```python
from build123d import *

# Parameters (mm, degrees)
SKETCH1_R                      = 6.35
SKETCH1_R_2                    = 5.08
BOSS_EXTRUDE1_DEPTH            = 15.494
BOSS_EXTRUDE2_DEPTH            = 13.462
SKETCH3_W                      = 1.016
SKETCH3_H                      = 0.508
BOSS_EXTRUDE3_DEPTH            = 1.27
SKETCH7_R                      = 1.397
CUT_EXTRUDE1_DEPTH             = 20.32
CUT_EXTRUDE4_REACH             = 23.971
CUT_EXTRUDE4_END_RADIUS        = 5.08
CUT_EXTRUDE4_DIRECTION_2_DEPTH = 0.635


with BuildPart() as part:
    # Sketch1 → Boss-Extrude1 (new body)
    with BuildSketch(Plane(origin=(0, 0, 0), x_dir=(0, 0, -1), z_dir=(1, 0, 0))):
        Circle(SKETCH1_R)
        Circle(SKETCH1_R_2, mode=Mode.SUBTRACT)
    extrude(amount=BOSS_EXTRUDE1_DEPTH)

    # Sketch2 → Boss-Extrude2 (add)
    with BuildSketch(Plane(origin=(1.016, 0, 0), x_dir=(0, 0, -1), z_dir=(1, 0, 0))):
        with BuildLine():
            Line((-2.0066, 6.024620854), (-2.0066, 14.224))
            Line((-2.0066, 14.224), (2.0066, 14.224))
            Line((2.0066, 14.224), (2.0066, 6.024620854))
            ThreePointArc((2.0066, 6.024620854), (0, 6.35), (-2.0066, 6.024620854))
        make_face()
    extrude(amount=BOSS_EXTRUDE2_DEPTH)

    # Sketch3 → Cut-Revolve1 (revolve, cut)
    with BuildSketch(Plane.XY, mode=Mode.PRIVATE) as cut_revolve1_sk:
        with Locations((14.986, 6.096)):
            Rectangle(SKETCH3_W, SKETCH3_H)
        with Locations((0.508, 6.096)):
            Rectangle(SKETCH3_W, SKETCH3_H)
    revolve(cut_revolve1_sk.sketch.rotate(Axis((15.494, 0, 0), (-1, 0, 0)), 90), axis=Axis((15.494, 0, 0), (-1, 0, 0)), mode=Mode.SUBTRACT)

    # Sketch5 → Boss-Extrude3 (add)
    with BuildSketch(Plane.ZY):
        with BuildLine():
            Line((4.709286039, 0.635), (4.709286039, -1.905))
            ThreePointArc((4.709286039, -1.905), (5.037440444, -0.656196444), (5.040156248, 0.635))
            Line((5.040156248, 0.635), (4.709286039, 0.635))
        make_face()
    extrude(amount=-BOSS_EXTRUDE3_DEPTH)

    # Sketch7 → Cut-Extrude1 (cut)
    with BuildSketch(Plane(origin=(0, -6.35, 0), x_dir=(1, 0, 0), z_dir=(0, 1, 0))):
        with Locations(Location((12.4206, 0, 0), (0, 0, 90))):
            Circle(SKETCH7_R)
        with Locations(Location((2.8956, 0, 0), (0, 0, 90))):
            Circle(SKETCH7_R)
        with Locations(Location((6.0706, 0, 0), (0, 0, 90))):
            Circle(SKETCH7_R)
        with Locations(Location((9.2456, 0, 0), (0, 0, 90))):
            Circle(SKETCH7_R)
    extrude(amount=CUT_EXTRUDE1_DEPTH, mode=Mode.SUBTRACT)

    # Cut-Extrude4: up to this cylinder (the profile starts inside it)
    cut_extrude4_end = Plane(origin=(0.846667, 0, 0), z_dir=(-1, 0, 0)) * Cylinder(CUT_EXTRUDE4_END_RADIUS, 59.102, mode=Mode.PRIVATE)
    # Sketch11 → Cut-Extrude4 (cut, up to the surface)
    with BuildSketch(Plane(origin=(0, 0, 0), x_dir=(1, 0, 0), z_dir=(0, 1, 0)), mode=Mode.PRIVATE) as cut_extrude4_sk1:
        Polygon((1.27, -4.709286039), (1.27, -5.040156248), (0, -4.709286039), align=None)
    cut_extrude4_tool1 = extrude(cut_extrude4_sk1.sketch, amount=-CUT_EXTRUDE4_REACH, mode=Mode.PRIVATE) & cut_extrude4_end
    add(cut_extrude4_tool1.solids().sort_by_distance((0.846667, 0, 4.819576))[0], mode=Mode.SUBTRACT)

    # Sketch11 → Cut-Extrude4 direction 2 (cut)
    with BuildSketch(Plane(origin=(0, 0, 0), x_dir=(1, 0, 0), z_dir=(0, 1, 0))):
        Polygon((1.27, -4.709286039), (1.27, -5.040156248), (0, -4.709286039), align=None)
    extrude(amount=CUT_EXTRUDE4_DIRECTION_2_DEPTH, mode=Mode.SUBTRACT)


solid = part.part
```
Verification items for the finished model (mm, model axes). A direction names the side the tool comes from. Coordinates: 2 decimals unless noted, no trailing zeros. Order: outer loops, then holes, each group sorted by start corner. A loop starts at its lowest first (then second) coordinate and runs counter-clockwise, first axis right, second up. Notation, with made-up numbers: (52.5, 34.5) - (83.5, 34.5) arc R18 cw to (83.5, 40.5) - close; hole circle Ø10 at (24.25, 0.5). An arc over 180 degrees is marked (long way). Return JSON: item names as keys, results as strings.
(1) Section check B-B, the plane z = -2.5. Record the cut outline in (x, y), and give its area (3 significant figures).
Filled sheet:
{"outline": "(0, -5.28) - (1.02, -5.28) - (1.02, -5.84) - (14.48, -5.84) - (14.48, -5.28) - (15.49, -5.28) - (15.49, -4.42) - (0, -4.42) - close; (0, 4.42) - (15.49, 4.42) - (15.49, 5.28) - (14.48, 5.28) - (14.48, 5.84) - (1.02, 5.84) - (1.02, 5.28) - (0, 5.28) - close", "area": "41.6 mm^2"}
(2) Access from +Z, -Z, +X, -X, +Y, -Y to the whole of each face (thin tool, end or side, straight path). Record for faces 1 (the flat face through (15.494, 5, 2)), 2 (the flat face through (14.478, 6, 0)), 3 (the cylindrical face through (7.434, 9.361, 0.303)), 4 (the flat face through (1.016, 6, 0)), 5 (the flat face through (8, 10, -2.007)).
Filled sheet:
{"face 1": "+Z, -Z, +X, +Y, -Y", "face 2": "+X", "face 3": "-Y", "face 4": "-X", "face 5": "-Z, +X, -X, +Y"}
(3) Go/stop test with flat-tipped pins: pin 1 (1.5 mm diameter, centred on y = -1.5, z = 2.5, fed in from -X); pin 2 (1.5 mm diameter, centred on x = 5.5, y = 5, fed in from -Z); pin 3 (1 mm diameter, centred on x = 6, z = -1, fed in from -Y); pin 4 (2.5 mm diameter, centred on x = 6.07, z = 0, fed in from -Y). Record where each tip stops, or that it passes through.
Filled sheet:
{"pin 1": "passes through", "pin 2": "stops at z = -4.72", "pin 3": "stops at y = -6.21", "pin 4": "stops at y = 13.97"}
(4) Thickness scan on line 1 along X through (y, z) = (-5.6, 0); line 2 along Z through (x, y) = (12.5, 8.5); line 3 along X through (y, z) = (9.25, -0.75). Record the ranges inside material, lowest first.
Filled sheet:
{"line 1": "x = 0 to 1.5, 4.29 to 4.67, 7.47 to 7.85, 10.64 to 11.02, 13.82 to 15.49", "line 2": "z = -2.01 to -1.39, 1.39 to 2.01", "line 3": "x = 1.02 to 1.72, 4.07 to 4.89, 7.25 to 8.07, 10.42 to 11.24, 13.6 to 14.48"}
(5) Section check D-D, the plane z = 0. Give the number of separate pieces and of enclosed holes in the cut face, and give its area (3 significant figures).
Filled sheet:
{"separate pieces": "6", "enclosed holes": "0", "area": "29.7 mm^2"}
(6) Section check C-C, the plane y = 9.25. Record the cut outline in (x, z), and give its area (3 significant figures).
Filled sheet:
{"outline": "(1.02, -2.01) - (14.48, -2.01) - (14.48, 2.01) - (1.02, 2.01) - close; hole circle Ø2.79 at (2.9, 0); hole circle Ø2.79 at (6.07, 0); hole circle Ø2.79 at (9.25, 0); hole circle Ø2.79 at (12.42, 0)", "area": "29.5 mm^2"}
(7) Mould release check, pull along X, two halves, no side actions. Record for faces 6 (the cylindrical face through (0.5, 3.6, 4.6)), 7 (the cylindrical face through (13.784, 9.361, 0.303)), 8 (the flat face through (3, 13.97, 0)), 9 (the flat face through (0.644, -0.371, 4.877)): pulls with the +X half, pulls with the -X half, needs draft (parallel to the pull), parting line crosses it, or undercut.
Filled sheet:
{"face 6": "needs draft", "face 7": "undercut", "face 8": "undercut", "face 9": "pulls with the +X half"}
